The listing builds one solid part. Answer for the finished solid, in the listing's coordinates (mm). A direction names the side the tool comes from. Round coordinates to 2 decimals unless told otherwise and drop trailing zeros. Order: outer loops, then holes, each group sorted by start corner. A loop starts at its lowest first (then second) coordinate and runs counter-clockwise, first axis right, second up. Notation, with made-up numbers: (40, -35) -> (97, -35) arc R30 ccw to (97, -6) -> close; hole circle Ø9 at (-37, -32.5). An arc over 180 degrees is marked (long way). Answer in a Markdown table with one row per item. Add a question column.
Autodesk Fusion 360 part; units mm, degrees
sketch "Skizze4" plane through (0, 0, 0) normal (0, 0, 1) x (1, 0, 0)
  line L0 (1.5, -6) -> (-1.5, -6)
  line L1 (-1.5, -6) -> (-1.5, 0)
  line L2 (-1.5, 0) -> (1.5, 0)
  line L3 (1.5, 0) -> (1.5, -6)
  line L4 (1.5, -6) -> (-1.5, 0) construction
  line L5 (-1.5, -6) -> (1.5, 0) construction
  line L6 (0, 9.7025) -> (0, -8.7035) construction
  line L7 (-7.2352, -6) -> (6.1757, -6) construction
  point P0 (0, -3)
  point P1 (0, -6)
  dimension "d21" = 3
  dimension "d22" = 6
ref_plane "Arbeitsebene1" through (0, 0, -6.5) normal (0, 0, 1) x (1, 0, 0)
sketch "Skizze7" plane through (0, 0, -6.5) normal (0, 0, 1) x (1, 0, 0)
  line L0 (-16.0259, 10) -> (20, 10) construction
  line L1 (-5, 21.68) -> (-5, -11.619) construction
  line L2 (5, 22.2413) -> (5, -12.5543) construction
  line L3 (-2.05, 11.7032) -> (-5, 13.4064)
  line L4 (-5, 13.4064) -> (-7.95, 11.7032)
  line L5 (-7.95, 11.7032) -> (-7.95, 8.2968)
  line L6 (-7.95, 8.2968) -> (-5, 6.5936)
  line L7 (-5, 6.5936) -> (-2.05, 8.2968)
  line L8 (-2.05, 8.2968) -> (-2.05, 11.7032)
  line L9 (7.95, 11.7032) -> (5, 13.4064)
  line L10 (5, 13.4064) -> (2.05, 11.7032)
  line L11 (2.05, 11.7032) -> (2.05, 8.2968)
  line L12 (2.05, 8.2968) -> (5, 6.5936)
  line L13 (5, 6.5936) -> (7.95, 8.2968)
  line L14 (7.95, 8.2968) -> (7.95, 11.7032)
  line L15 (-15.7752, 15) -> (18.7006, 15) construction
  line L16 (0, 22.633) -> (0, -9.7229) construction
  line L17 (2.95, 16.7032) -> (0, 18.4064)
  line L18 (0, 18.4064) -> (-2.95, 16.7032)
  line L19 (-2.95, 16.7032) -> (-2.95, 13.2968)
  line L20 (-2.95, 13.2968) -> (0, 11.5936)
  line L21 (0, 11.5936) -> (2.95, 13.2968)
  line L22 (2.95, 13.2968) -> (2.95, 16.7032)
  point P0 (-5, 10)
  point P1 (5, 10)
  point P2 (-5, 10)
  point P3 (5, 10)
  point P4 (0, 15)
  point P5 (0, 15)
  dimension "d47" = 5.9
  dimension "d48" = 5.9
  dimension "d51" = 15
  dimension "d52" = 5.9
  dimension "d117" = 10
  dimension "d118" = 5
  dimension "d119" = 5
sketch "Skizze1" plane through (0, 0, 0) normal (1, 0, 0) x (0, 1, 0) in component "Unterteil"
  line L0 (0, 9.24) -> (0, -14) construction
  line L1 (-13.3055, 0) -> (32, 0) construction
  line L2 (-6, -10) -> (20, -10)
  line L3 (20, -10) -> (20, 0)
  line L4 (90, 0) -> (90, -15)
  line L5 (90, -15) -> (-6, -15)
  line L6 (-6, -15) -> (-6, -10)
  line L7 (90, 0) -> (20, 0)
  line L8 (25, 1.4735) -> (25, -18) construction
  line L9 (33.3576, -5) -> (21.4671, -5) construction
  circle A0 centre (25, -5) radius 4.1
  dimension "d60" = 70
  dimension "d61" = 15
  dimension "d64" = 8.2
  dimension "d120" = 25
  dimension "d121" = 5
  dimension "d122" = 15
  dimension "d123" = 10
  dimension "d124" = 20
  dimension "d125" = 6
extrude "Extrusion1" add sketch "Skizze1" along normal mid plane 20 in component "Unterteil"
sketch "Skizze2" plane through (0, 0, -15) normal (0, 0, -1) x (1, 0, 0) in component "Unterteil"
  line L0 (-10, -90) -> (10, -90)
  line L1 (10, -90) -> (10, 6)
  line L2 (10, 6) -> (-10, 6)
  line L3 (-10, 6) -> (-10, -90)
  line L4 (14.3477, -10) -> (-22.3478, -10) construction
  line L5 (5, -37) -> (5, 12.4856) construction
  line L6 (-5, -37.5119) -> (-5, 12) construction
  circle A0 centre (-5, -10) radius 1.75
  circle A1 centre (5, -10) radius 1.75
  circle A2 centre (5, -10) radius 3.5
  circle A3 centre (-5, -10) radius 3.5
  dimension "d67" = 16
  dimension "d68" = 5
  dimension "d69" = 5
  dimension "d70" = 3.5
  dimension "d71" = 3.5
  dimension "d72" = 7
  dimension "d73" = 7
extrude "Extrusion2" cut sketch "Skizze2" against normal blind 10 contours A0 | A1 in component "Unterteil"
extrude "Extrusion3" cut sketch "Skizze2" against normal blind 2 contours A2 | A3 in component "Unterteil"
fillet "Abrundung3" radius 5 1 edges at (0, -6, -15) in component "Unterteil"
fillet "Abrundung4" radius 5 1 edges at (0, 90, 0) in component "Unterteil"
fillet "Abrundung5" radius 5 1 edges at (0, 90, -15) in component "Unterteil"
component "Unterteil" placed x (1, 0, 0) y (0, 1, 0) z (0, 0, 1) at (0, 0, 0)
component "Basis" placed x (1, 0, 0) y (0, 1, 0) z (0, 0, 1) at (0, 0, 0)
1. For faces 1 (the flat face through (0, 20, -5)), 2 (the cylindrical face through (-5.759, 13.417, -14.014)), 3 (the flat face through (10, 52, -7)), determine the directions among +Z, -Z, +X, -X, +Y, -Y from which every point of the face is accessible in a straight line to the end or side of a thin tool.
2. Straight lines are drawn through the part: line 1 along X through (y, z) = (10, -11.2); line 2 along X through (y, z) = (10, -14.3); line 3 along Z through (x, y) = (-2.5, 25). For each, find the intervals that lie inside material, in ascending order.
3. The mould has two halves that part along Y. Classify faces 4 (the flat face through (6, 8, -13)), 5 (the cylindrical face through (8.233, 11.341, -14.014)), 6 (the cylindrical face through (0, -5, -13)), 7 (the flat face through (0, 7, -10)): released by +Y, released by -Y, zero draft, split by the parting line, or undercut.
4. Each of these flat-tipped pins is pushed along its axis until it touches: pin 1 (6 mm diameter, centred on x = 4.5, z = -11, fed in from -Y); pin 2 (8 mm diameter, centred on x = -5, y = 10, fed in from +Z); pin 3 (5 mm diameter, centred on x = 1.5, z = -6.5, fed in from -Y); pin 4 (2 mm diameter, centred on x = -6, y = 11.5, fed in from -Z). Where does it stop, or does it pass through?
5. The part is cut by section C-C (z = -3). Give the vertices of the cut face in (x, y).
6. The part is cut by section A-A (x = -5). Give the number of separate pieces and of enclosed holes in the cut face, then the cut area to 3 significant figures.
7. The part is cut by section B-B (y = 25). Give the vertices of the cut face in (x, z), then the cut area to 3 significant figures.
8. The part is cut by section D-D (y = 10). Give the vertices of the cut face in (x, z).
Report:
| question | item | result |
|---|---|---|
| 1 | face 1 | +Z, +X, -X, -Y |
| 1 | face 2 | -Z |
| 1 | face 3 | +Z, -Z, +X, +Y, -Y |
| 2 | line 1 | x = -10 to -6.75, -3.25 to 3.25, 6.75 to 10 |
| 2 | line 2 | x = -10 to -8.5, -1.5 to 1.5, 8.5 to 10 |
| 2 | line 3 | z = -15 to -9.1, -0.9 to 0 |
| 3 | face 4 | undercut |
| 3 | face 5 | undercut |
| 3 | face 6 | released by -Y |
| 3 | face 7 | zero draft |
| 4 | pin 1 | stops at y = -6 |
| 4 | pin 2 | stops at z = -10 |
| 4 | pin 3 | stops at y = 20 |
| 4 | pin 4 | stops at z = -13 |
| 5 | outline | (-10, 20) -> (10, 20) -> (10, 21.42) -> (-10, 21.42) -> close; (-10, 28.58) -> (10, 28.58) -> (10, 89.58) -> (-10, 89.58) -> close |
| 6 | separate pieces | 2 |
| 6 | enclosed holes | 1 |
| 6 | area | 1,090 mm^2 |
| 7 | outline | (-10, -15) -> (10, -15) -> (10, -9.1) -> (-10, -9.1) -> close; (-10, -0.9) -> (10, -0.9) -> (10, 0) -> (-10, 0) -> close |
| 7 | area | 136 mm^2 |
| 8 | outline | (-10, -15) -> (-8.5, -15) -> (-8.5, -13) -> (-6.75, -13) -> (-6.75, -10) -> (-10, -10) -> close; (-3.25, -13) -> (-1.5, -13) -> (-1.5, -15) -> (1.5, -15) -> (1.5, -13) -> (3.25, -13) -> (3.25, -10) -> (-3.25, -10) -> close; (6.75, -13) -> (8.5, -13) -> (8.5, -15) -> (10, -15) -> (10, -10) -> (6.75, -10) -> close |
